from build123d import *

# Parameters (mm, degrees)
SKETCH1_W           = 5
SKETCH1_H           = 22
BOSS_EXTRUDE1_DEPTH = 150
CUT_EXTRUDE1_DEPTH  = 161.573187019
CUT_EXTRUDE2_DEPTH  = 161.573187019
SKETCH4_W           = 5
SKETCH4_H           = 6
BOSS_EXTRUDE2_DEPTH = 3
SKETCH5_W           = 5
SKETCH5_H           = 6
BOSS_EXTRUDE3_DEPTH = 3
SKETCH6_W           = 30
SKETCH6_H           = 5
BOSS_EXTRUDE4_DEPTH = 5
SKETCH7_W           = 5
SKETCH7_H           = 5
CUT_EXTRUDE3_DEPTH  = 166.192623536
SKETCH8_W           = 5
SKETCH8_H           = 5
CUT_EXTRUDE4_DEPTH  = 166.192623536


with BuildPart() as part:
    # Sketch1 → Boss-Extrude1 (new body)
    with BuildSketch(Plane.XY):
        with Locations((31.394042166, 46.08544814)):
            Rectangle(SKETCH1_W, SKETCH1_H)
    extrude(amount=BOSS_EXTRUDE1_DEPTH)

    # Sketch2 → Cut-Extrude1 (cut, through all)
    with BuildSketch(Plane(origin=(33.894042166, 0, 0), x_dir=(0, 0, -1), z_dir=(1, 0, 0))):
        with BuildLine():
            Line((-93, 49.08544814), (-57, 49.08544814))
            ThreePointArc((-57, 49.08544814), (-54.171572875, 47.913875265), (-53, 45.08544814))
            Line((-53, 45.08544814), (-29, 45.08544814))
            ThreePointArc((-29, 45.08544814), (-21.928932188, 42.156515952), (-19, 35.08544814))
            Line((-19, 35.08544814), (-131, 35.08544814))
            ThreePointArc((-131, 35.08544814), (-128.071067812, 42.156515952), (-121, 45.08544814))
            Line((-121, 45.08544814), (-97, 45.08544814))
            ThreePointArc((-97, 45.08544814), (-95.828427125, 47.913875265), (-93, 49.08544814))
        make_face()
    extrude(amount=-CUT_EXTRUDE1_DEPTH, mode=Mode.SUBTRACT)

    # Sketch3 → Cut-Extrude2 (cut, through all)
    with BuildSketch(Plane(origin=(33.894042166, 0, 0), x_dir=(0, 0, -1), z_dir=(1, 0, 0))):
        Polygon((-38.5, 51.08544814), (-35.5, 51.08544814), (-35.5, 52.53544814), (-34.25, 52.53544814), (-34.25, 55.08544814), (-35.5, 55.08544814), (-35.5, 57.08544814), (-38.5, 57.08544814), (-38.5, 55.08544814), (-39.75, 55.08544814), (-39.75, 52.53544814), (-38.5, 52.53544814), align=None)
        Polygon((-111.5, 57.08544814), (-114.5, 57.08544814), (-114.5, 55.08544814), (-115.75, 55.08544814), (-115.75, 52.53544814), (-114.5, 52.53544814), (-114.5, 51.08544814), (-111.5, 51.08544814), (-111.5, 52.53544814), (-110.25, 52.53544814), (-110.25, 55.08544814), (-111.5, 55.08544814), align=None)
        Polygon((-10, 44.58544814), (-4.55, 44.58544814), (-4.55, 43.33544814), (-2, 43.33544814), (-2, 44.58544814), (0, 44.58544814), (0, 47.58544814), (-2, 47.58544814), (-2, 48.83544814), (-4.55, 48.83544814), (-4.55, 47.58544814), (-10, 47.58544814), align=None)
        Polygon((-145.45, 47.58544814), (-145.45, 48.83544814), (-148, 48.83544814), (-148, 47.58544814), (-150, 47.58544814), (-150, 44.58544814), (-148, 44.58544814), (-148, 43.33544814), (-145.45, 43.33544814), (-145.45, 44.58544814), (-140, 44.58544814), (-140, 47.58544814), align=None)
    extrude(amount=-CUT_EXTRUDE2_DEPTH, mode=Mode.SUBTRACT)

    # Sketch4 → Boss-Extrude2 (add)
    with BuildSketch(Plane(origin=(0, 0, 0), x_dir=(-1, 0, 0), z_dir=(0, 0, -1))):
        with Locations((-31.394042166, 38.08544814)):
            Rectangle(SKETCH4_W, SKETCH4_H)
        with Locations((-31.394042166, 54.08544814)):
            Rectangle(SKETCH4_W, SKETCH4_H)
    extrude(amount=BOSS_EXTRUDE2_DEPTH)

    # Sketch5 → Boss-Extrude3 (add)
    with BuildSketch(Plane.XY.offset(150)):
        with Locations((31.394042166, 54.08544814)):
            Rectangle(SKETCH5_W, SKETCH5_H)
        with Locations((31.394042166, 38.08544814)):
            Rectangle(SKETCH5_W, SKETCH5_H)
    extrude(amount=BOSS_EXTRUDE3_DEPTH)

    # Sketch6 → Boss-Extrude4 (add)
    with BuildSketch(Plane(origin=(33.894042166, 0, 0), x_dir=(0, 0, -1), z_dir=(1, 0, 0))):
        with Locations((-75, 59.58544814)):
            Rectangle(SKETCH6_W, SKETCH6_H)
    extrude(amount=-BOSS_EXTRUDE4_DEPTH)

    # Sketch7 → Cut-Extrude3 (cut, through all)
    with BuildSketch(Plane.ZY.offset(-28.894042166)):
        with Locations((123.5, 54.58544814)):
            Rectangle(SKETCH7_W, SKETCH7_H)
        with Locations((26.5, 54.58544814)):
            Rectangle(SKETCH7_W, SKETCH7_H)
    extrude(amount=-CUT_EXTRUDE3_DEPTH, mode=Mode.SUBTRACT)

    # Sketch8 → Cut-Extrude4 (cut, through all)
    with BuildSketch(Plane.ZY.offset(-28.894042166)):
        with Locations((47.5, 54.58544814)):
            Rectangle(SKETCH8_W, SKETCH8_H)
        with Locations((102.5, 54.58544814)):
            Rectangle(SKETCH8_W, SKETCH8_H)
    extrude(amount=-CUT_EXTRUDE4_DEPTH, mode=Mode.SUBTRACT)


solid = part.part
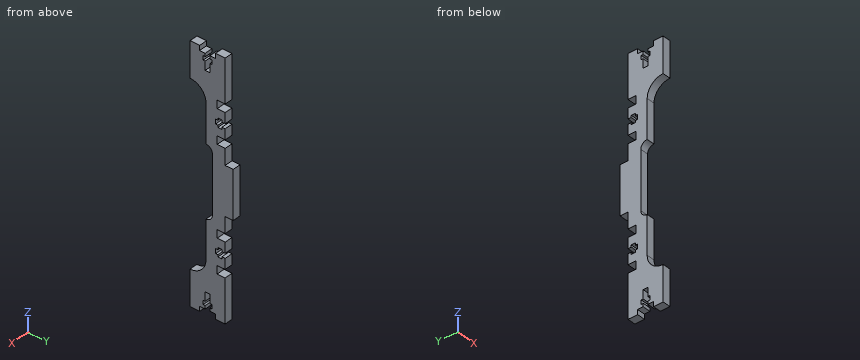
Design review of the part built by this model. Coordinates are the model's own, in mm. Give positions to 0.01 mm unless a question says otherwise; leave off trailing zeros. Write each loop counter-clockwise with the first axis right and the second up, starting at its lowest first coordinate (ties: lowest second). Pieces come first, ordered by that corner, then holes. Notation, with made-up numbers: M 77,46.25 L 89,46.25 A24 ccw 89,81.25 Z; hole C 79,-8.5 d4. An arc over 180 degrees is marked long. Answer as a JSON object with one key per item and string values. Group by question number.
1) We need section A-A (z = 103). Give the boundary of the cut face in (x, y).
2) For line 1 along Y through (x, z) = (29.4, 141); line 2 along Y through (x, z) = (33.05, 111); line 3 along Y through (x, z) = (32.8, 78), list the stretches that pass through material, from the lowest coordinate up.
3) Clearance check with flat-ended pins moving along their axes: pin 1 Ø8 at (y, z) = (41, 117.5) entering from +X; pin 2 Ø1 at (x, z) = (29.5, 109) entering from -Y; pin 3 Ø1.3 at (x, z) = (32.5, 3.5) entering from +Y; pin 4 Ø1 at (x, y) = (30.5, 44) entering from +Z. State where each tip first meets the part, or that it passes through.
4) We need section B-B (z = 138). Give the boundary of the cut face in (x, y), and give its area (3 significant figures).
Answer key:
{
 "1": {"outline": "M 28.89,45.09 L 33.89,45.09 L 33.89,52.09 L 28.89,52.09 Z"},
 "2": {"line 1": "y = 35.09 to 44.59, 47.59 to 57.09", "line 2": "y = 45.09 to 52.54, 55.09 to 57.09", "line 3": "y = 49.09 to 62.09"},
 "3": {"pin 1": "passes through", "pin 2": "stops at y = 45.09", "pin 3": "stops at y = 57.09", "pin 4": "stops at z = 150"},
 "4": {"outline": "M 28.89,35.09 L 33.89,35.09 L 33.89,57.09 L 28.89,57.09 Z", "area": "110 mm²"}
}
